```python
from build123d import *

# Parameters (mm, degrees)
SKETCH1_W           = 265
SKETCH1_H           = 180
BOSS_EXTRUDE1_DEPTH = 10
BOSS_EXTRUDE2_START = -17
BOSS_EXTRUDE2_DEPTH = 17
FILLET1_R           = 6
FILLET2_R           = 6
CUT_EXTRUDE2_START  = -265
CUT_EXTRUDE2_DEPTH  = 265


# Read off the part's stored shape, not the designer's step: Boss-Extrude2, Cut-Extrude2
with BuildPart() as part:
    # Sketch1 → Boss-Extrude1 (new body)
    with BuildSketch(Plane.XY):
        Rectangle(SKETCH1_W, SKETCH1_H)
    extrude(amount=BOSS_EXTRUDE1_DEPTH)

    # Boss-Extrude2 outline → Boss-Extrude2 (add)
    with BuildSketch(Plane.ZY.offset(132.5).offset(BOSS_EXTRUDE2_START)):
        with BuildLine():
            ThreePointArc((0, -81.626136458), (-13.387109794, -89.880720577), (1.939630355, -93.408312392))
            add(Edge.make_bspline(
                [(1.939630355, -93.408312392), (5.863215247, -91.451215581), (10, -90)],
                knots=[0, 0, 0, 1, 1, 1], degree=2))
            Line((10, -90), (0, -90))
            Line((0, -90), (0, -81.626136458))
        make_face()
    boss_extrude2 = extrude(amount=BOSS_EXTRUDE2_DEPTH)

    # Mirror1: Boss-Extrude2 across plane
    add(boss_extrude2.mirror(Plane(origin=(0, 0, 0), x_dir=(0, 0, 1), z_dir=(1, 0, 0))))

    # Fillet1
    fillet1_edges = [part.edges().sort_by_distance(p)[0] for p in [
        (132.5, 0, 10),
        (0, 90, 10),
        (-132.5, 0, 10),
    ]]
    fillet(fillet1_edges, radius=FILLET1_R)

    # Fillet2
    fillet2_edges = [part.edges().sort_by_distance(p)[0] for p in [
        (0, -90, 10),
    ]]
    fillet(fillet2_edges, radius=FILLET2_R)

    # Cut-Extrude2 outline → Cut-Extrude2 (cut)
    with BuildSketch(Plane.ZY.offset(132.5).offset(CUT_EXTRUDE2_START)):
        with BuildLine():
            add(Edge.make_bspline(
                [(1.939630355, -93.408312392), (2.161603751, -91.034387849), (4, -90)],
                knots=[0, 0, 0, 1, 1, 1], degree=2))
            add(Edge.make_bspline(
                [(1.939630355, -93.408312392), (5.863215247, -91.451215581), (10, -90)],
                knots=[0, 0, 0, 1, 1, 1], degree=2))
            Line((10, -90), (10, -84))
            ThreePointArc((10, -84), (8.242640687, -88.242640687), (4, -90))
        make_face()
    extrude(amount=CUT_EXTRUDE2_DEPTH, mode=Mode.SUBTRACT)


solid = part.part
```
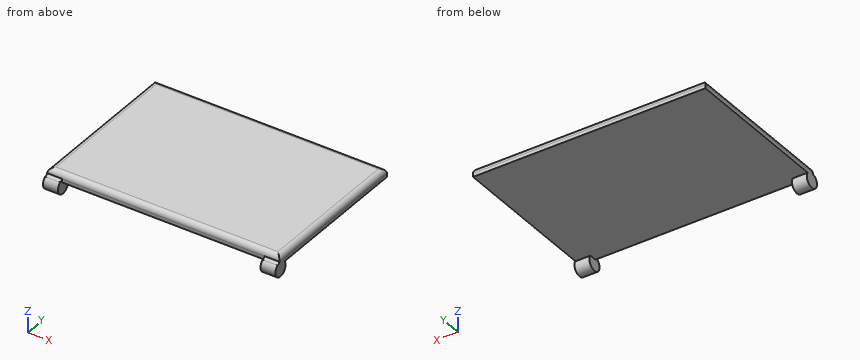
Geometry: final body of the model. Coordinates: model frame, mm. Give positions to 0.01 mm unless a question says otherwise; leave off trailing zeros. Loops run counter-clockwise (first coordinate to the right, second up) from the corner with the lowest first, then second, coordinate; pieces in that order, holes last. Notation, with made-up numbers: (14, 49.5) -> (41, 49.5) arc R30 ccw to (41, 85.5) -> close; hole circle Ø4 at (-6.5, 89). An arc over 180 degrees is marked (long way). Use CSV: the item, a comma, the result in double quotes.
(1) Ray query, line 1 along X through (y, z) = (-85, -7.5); line 2 along Z through (x, y) = (82, 66); line 3 along Y through (x, z) = (28, 1.25). Return the intervals inside material, ascending. Write a range as [from, to].
From the geometry:
line 1,"[-132.5, -115.5], [115.5, 132.5]"
line 2,"[0, 10]"
line 3,"[-90, 90]"
(2) Cut plane D-D (z = 7.25). Output: boundary loops of the cut face in (x, y), plus the area to 3 significant figures.
From the geometry:
outline,"(-131.54, -89.04) -> (131.54, -89.04) -> (131.54, 89.04) -> (-131.54, 89.04) -> close"
area,"46,900 mm^2"
(3) Cut plane A-A (z = -5). Output: boundary loops of the cut face in (x, y).
From the geometry:
outline,"(-132.5, -97) -> (-115.5, -97) -> (-115.5, -80) -> (-132.5, -80) -> close; (115.5, -97) -> (132.5, -97) -> (132.5, -80) -> (115.5, -80) -> close"
(4) Cut plane C-C (y = 15). Output: boundary loops of the cut face in (x, z).
From the geometry:
outline,"(-132.5, 0) -> (132.5, 0) -> (132.5, 4) arc R6 ccw to (126.5, 10) -> (-126.5, 10) arc R6 ccw to (-132.5, 4) -> close"
(5) Cut plane B-B (x = -108). Output: boundary loops of the cut face in (y, z).
From the geometry:
outline,"(-90, 0) -> (90, 0) -> (90, 4) arc R6 ccw to (84, 10) -> (-84, 10) arc R6 ccw to (-90, 4) -> close"
(6) First-contact query: P1, Ø2, axis at x = 14, y = -38.5, coming from the -Z side; P2, Ø2, axis at y = -34, z = 7, coming from the -X side; P3, Ø3, axis at x = -55, z = 2, coming from the -Y side. Flat tips, straight axial feed; report the tip coordinate or a pass-through.
From the geometry:
P1,"z = 0"
P2,"x = -132.16"
P3,"y = -90"
